The listing builds one solid part. Answer for the finished solid, in the listing's coordinates (mm). Face numbers are marked on the shaded views. A direction names the side the tool comes from. Coordinates: 2 decimals unless noted, no trailing zeros. Order: outer loops, then holes, each group sorted by start corner. A loop starts at its lowest first (then second) coordinate and runs counter-clockwise, first axis right, second up. Notation, with made-up numbers: (-32, 55.25) -> (25, 55.25) arc R23 cw to (25, 63.25) -> close; hole circle Ø6 at (86.25, 39). An arc over 180 degrees is marked (long way). Return JSON: item names as keys, results as strings.
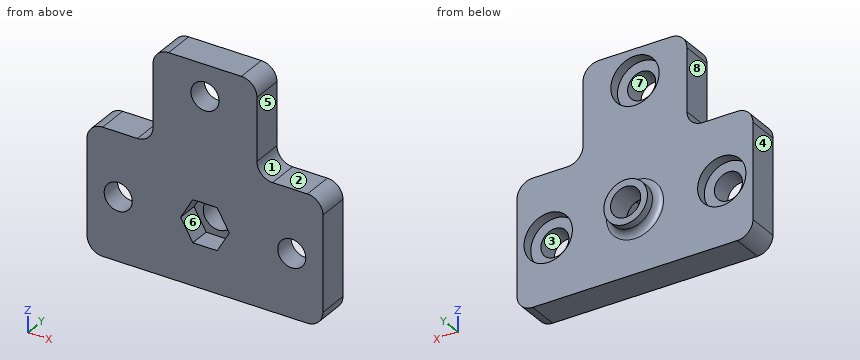
Autodesk Inventor part; units mm, degrees
ref_plane "YZ Plane" through (0, 0, 0) normal (1, 0, 0) x (0, 1, 0)
ref_plane "XZ Plane" through (0, 0, 0) normal (0, 1, 0) x (-1, 0, 0)
ref_plane "XY Plane" through (0, 0, 0) normal (0, 0, 1) x (1, 0, 0)
sketch "Boceto1" plane through (0, 0, 0) normal (0, 1, 0) x (-1, 0, 0)
  circle A0 centre (0, 0) radius 12.15
  dimension "d0" = 24.3
extrude "Extrusión1" add sketch "Boceto1" along normal blind 4
sketch "Boceto2" plane through (0, 0, 0) normal (0, -1, 0) x (1, 0, 0)
  line L0 (4.6765, 0) -> (2.3383, -4.05)
  line L1 (2.3383, -4.05) -> (-2.3383, -4.05)
  line L2 (-2.3383, -4.05) -> (-4.6765, 0)
  line L3 (-4.6765, 0) -> (-2.3383, 4.05)
  line L4 (-2.3383, 4.05) -> (2.3383, 4.05)
  line L5 (2.3383, 4.05) -> (4.6765, 0)
  circle A0 centre (0, 0) radius 4.05
  dimension "d3" = 8.1
extrude "Extrusión2" cut sketch "Boceto2" against normal blind 4
sketch "Boceto3" plane through (0, 4, 0) normal (0, 1, 0) x (1, 0, 0)
  line L0 (2.3383, 4.05) -> (4.6765, 0)
  line L1 (4.6765, 0) -> (2.3383, -4.05)
  line L2 (2.3383, -4.05) -> (-2.3383, -4.05)
  line L3 (-2.3383, -4.05) -> (-4.6765, 0)
  line L4 (-4.6765, 0) -> (-2.3383, 4.05)
  line L5 (-2.3383, 4.05) -> (2.3383, 4.05)
  circle A0 centre (0, 0) radius 12.15
  circle A1 centre (0, 0) radius 2.9
  dimension "d6" = 5.8
extrude "Extrusión3" add sketch "Boceto3" along normal blind 2 contours L0 L1 L2 L3 L4 L5 | A0
sketch "Boceto4" plane through (0, 6, 0) normal (0, 1, 0) x (1, 0, 0)
  circle A0 centre (0, 0) radius 4.2
  circle A1 centre (0, 0) radius 2.9
  dimension "d9" = 8.4
extrude "Extrusión4" add sketch "Boceto4" along normal blind 2.8
fillet "Empalme1" radius 1.3 1 edges at (-4.2, 6, 0)
sketch "Boceto5" plane through (0, 6, 0) normal (0, 1, 0) x (1, 0, 0)
  line L0 (-22.7, -12.15) -> (22.7, -12.15)
  line L1 (22.7, -12.15) -> (22.7, 12.15)
  line L2 (22.7, 12.15) -> (-22.7, 12.15)
  line L3 (-22.7, 12.15) -> (-22.7, -12.15)
  circle A0 centre (0, 0) radius 2.9
  line L4 (-22.7, -12.15) -> (22.7, 12.15) construction
  line L5 (22.7, -12.15) -> (-22.7, 12.15) construction
  circle A1 centre (0, 0) radius 12.15
  point P0 (0, -12.15)
  point P1 (0, 12.15)
  dimension "d13" = 45.4
extrude "Extrusión5" add sketch "Boceto5" against normal up to surface (6 mm away) contours L3 L2 A1 L0 | A1 L2 L1 L0
sketch "Boceto6" plane through (0, 6, 0) normal (0, 1, 0) x (1, 0, 0)
  circle A0 centre (-16.7, 0) radius 2.7
  circle A1 centre (16.7, 0) radius 2.7
  line L0 (-22.7, 12.15) -> (-22.7, -12.15)
  line L1 (22.7, -12.15) -> (22.7, 12.15)
  point P0 (0, 0)
  dimension "d16" = 5.4
  dimension "d17" = 6
  dimension "d18" = 6
extrude "Extrusión6" cut sketch "Boceto6" against normal through all
fillet "Empalme2" radius 3 4 edges at (-22.7, 3, 12.15) (22.7, 3, 12.15) (-22.7, 3, -12.15) (22.7, 3, -12.15)
sketch "Boceto7" plane through (0, 6, 0) normal (0, 1, 0) x (1, 0, 0)
  line L0 (-10, 30.2) -> (10, 30.2)
  line L1 (10, 30.2) -> (10, -30.2)
  line L2 (10, -30.2) -> (-10, -30.2)
  line L3 (-10, -30.2) -> (-10, 30.2)
  line L4 (-10, 30.2) -> (10, -30.2) construction
  line L5 (10, 30.2) -> (-10, -30.2) construction
  line L6 (-19.7, -12.15) -> (19.7, -12.15)
  circle A0 centre (0, -24.2) radius 2.7
  circle A1 centre (0, 0) radius 21.5
  point P0 (10, -12.15)
  point P1 (-10, -12.15)
  dimension "d22" = 20
  dimension "d24" = 5.4
  dimension "d25" = 6
  dimension "d29" = 43
extrude "Extrusión7" add sketch "Boceto7" against normal up to surface (6 mm away) contours L6 L1 A1 L3 | A1 L1 L2 L3 picked at (0, -15.2667)
fillet "Empalme3" radius 3 4 edges at (-10, 3, 12.15) (-10, 3, 30.2) (10, 3, 30.2) (10, 3, 12.15)
sketch "Boceto9" plane through (0, 6, 0) normal (0, 1, 0) x (1, 0, 0)
  circle A0 centre (16.7, 0) radius 2.7
  circle A1 centre (16.7, 0) radius 4.65
  circle A2 centre (-16.7, 0) radius 2.7
  circle A3 centre (-16.7, 0) radius 4.65
  circle A4 centre (0, -24.2) radius 2.7
  circle A5 centre (0, -24.2) radius 4.65
  point P0 (0, 0)
  dimension "d30" = 9.3
extrude "Extrusión8" cut sketch "Boceto9" against normal blind 2 contours A0 | A1 | A2 | A3 | A4 | A5
sketch "Boceto10" plane through (0, 6, 0) normal (0, 1, 0) x (1, 0, 0)
  circle A0 centre (0, 0) radius 2.9
  circle A1 centre (0, 0) radius 12
  dimension "d33" = 24
properties part number "Pulley support"
1. Determine the mould class of the marked faces 1, 2, 3 and 4 for opening direction X: pulls with the +X half, pulls with the -X half, needs draft (parallel to the pull), parting line crosses it, or undercut.
Answer block:
{"face 1": "pulls with the +X half", "face 2": "needs draft", "face 3": "undercut", "face 4": "pulls with the -X half"}
2. The part is cut by section D-D on x = 16.7. Give the vertices of the cut face in (y, z).
Answer block:
{"outline": "(0, -12.15) -> (6, -12.15) -> (6, -4.65) -> (4, -4.65) -> (4, -2.7) -> (0, -2.7) -> close; (0, 2.7) -> (4, 2.7) -> (4, 4.65) -> (6, 4.65) -> (6, 12.15) -> (0, 12.15) -> close"}
3. Consider line 1 (X direction, y = 4.7, z = 0); line 2 (Z direction, x = 0, y = 5.6); line 3 (Z direction, x = 0, y = 1.8). Determine where each line is inside the solid, lowest interval first. Write a range as from..to.
Answer block:
{"line 1": "x = -22.7..-21.35, -12.05..-2.9, 2.9..12.05, 21.35..22.7", "line 2": "z = -12.15..-2.9, 2.9..19.55, 28.85..30.2", "line 3": "z = -12.15..-4.05, 4.05..21.5, 26.9..30.2"}
4. The part is cut by section C-C on z = 24.2. Give the vertices of the cut face in (x, y), and give its area (3 significant figures).
Answer block:
{"outline": "(-10, 0) -> (-2.7, 0) -> (-2.7, 4) -> (-4.65, 4) -> (-4.65, 6) -> (-10, 6) -> close; (2.7, 0) -> (10, 0) -> (10, 6) -> (4.65, 6) -> (4.65, 4) -> (2.7, 4) -> close", "area": "79.8 mm2"}
5. Each of these flat-tipped pins is pushed along its axis until it touches: pin 1 Ø10.5 at (x, z) = (0, 24.2) entering from +Y; pin 2 Ø3 at (x, y) = (-15.5, 2.5) entering from +Z; pin 3 Ø4.5 at (x, z) = (-16.5, -1.5) entering from +Y. Where does it stop, or does it pass through?
Answer block:
{"pin 1": "stops at y = 6", "pin 2": "stops at z = 12.15", "pin 3": "stops at y = 4"}
6. The part is cut by section A-A on y = 3. Give the vertices of the cut face in (x, z).
Answer block:
{"outline": "(-22.7, -9.15) arc R3 ccw to (-19.7, -12.15) -> (19.7, -12.15) arc R3 ccw to (22.7, -9.15) -> (22.7, 9.15) arc R3 ccw to (19.7, 12.15) -> (13, 12.15) arc R3 cw to (10, 15.15) -> (10, 27.2) arc R3 ccw to (7, 30.2) -> (-7, 30.2) arc R3 ccw to (-10, 27.2) -> (-10, 15.15) arc R3 cw to (-13, 12.15) -> (-19.7, 12.15) arc R3 ccw to (-22.7, 9.15) -> close; hole circle Ø5.4 at (-16.7, 0); hole (-4.68, 0) -> (-2.34, -4.05) -> (2.34, -4.05) -> (4.68, 0) -> (2.34, 4.05) -> (-2.34, 4.05) -> close; hole circle Ø5.4 at (0, 24.2); hole circle Ø5.4 at (16.7, 0)"}
7. For the marked faces 5, 6, 7 and 8, determine the directions among +Z, -Z, +X, -X, +Y, -Y from which every point of the face is accessible in a straight line to the end or side of a thin tool.
Answer block:
{"face 5": "+Z, +X, +Y, -Y", "face 6": "-Y", "face 7": "+Y, -Y", "face 8": "+Z, -X, +Y, -Y"}
8. The part is cut by section B-B on x = 0. Give the vertices of the cut face in (y, z), and give its area (3 significant figures).
Answer block:
{"outline": "(0, -12.15) -> (6, -12.15) -> (6, -5.5) arc R1.3 cw to (7.3, -4.2) -> (8.8, -4.2) -> (8.8, -2.9) -> (4, -2.9) -> (4, -4.05) -> (0, -4.05) -> close; (0, 4.05) -> (4, 4.05) -> (4, 2.9) -> (8.8, 2.9) -> (8.8, 4.2) -> (7.3, 4.2) arc R1.3 cw to (6, 5.5) -> (6, 19.55) -> (4, 19.55) -> (4, 21.5) -> (0, 21.5) -> close; (0, 26.9) -> (4, 26.9) -> (4, 28.85) -> (6, 28.85) -> (6, 30.2) -> (0, 30.2) -> close", "area": "178 mm2"}
